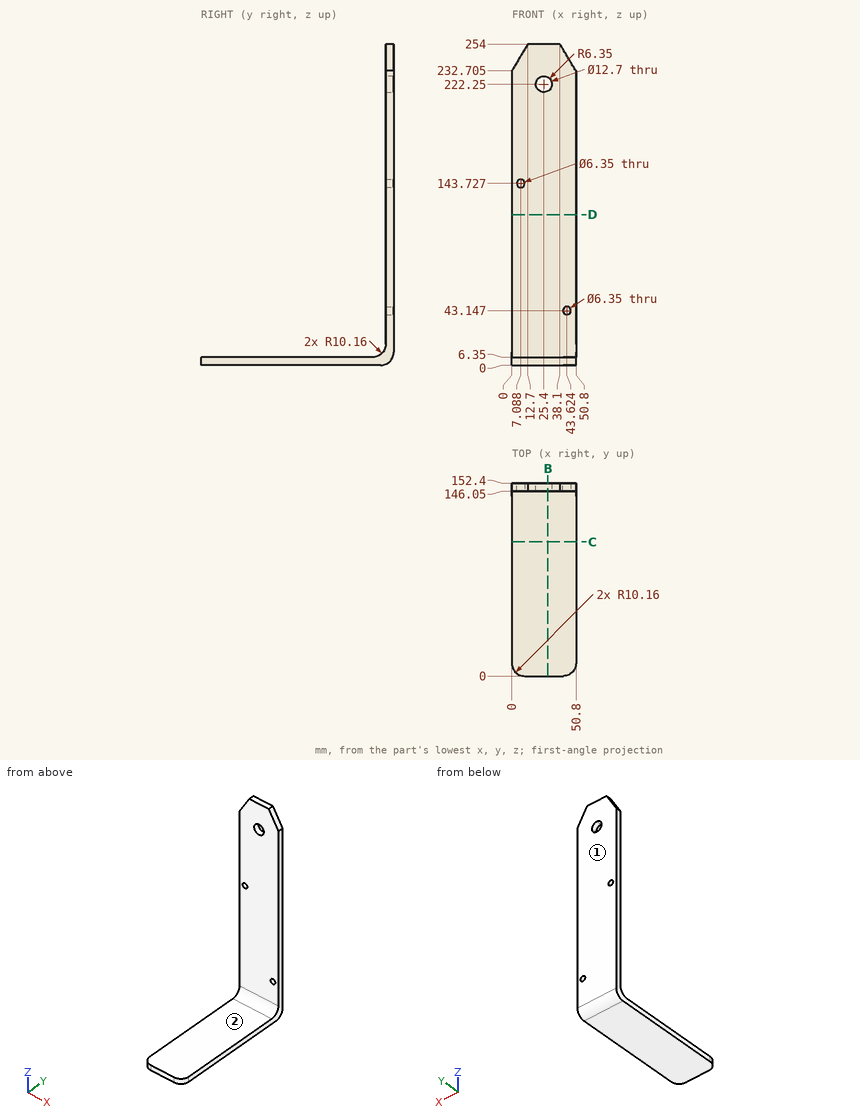
For this review, use the dimensioned drawing (mm, ordinates from the lowest corner) and the shaded views. A direction names the side the tool comes from. Coordinates: 2 decimals unless noted, no trailing zeros. Order: outer loops, then holes, each group sorted by start corner. A loop starts at its lowest first (then second) coordinate and runs counter-clockwise, first axis right, second up. Notation, with made-up numbers: (-21.5, -35) - (-8.5, -35) arc R15 cw to (-8.5, -19) - close; hole circle Ø3 at (22, 1.5). An arc over 180 degrees is marked (long way). Answer as a JSON object with one key per item and string values. Group by question number.
1. Clearance check with flat-ended pins moving along their axes: P1, Ø12, axis at x = 18.5, y = 119, coming from the +Z side; P2, Ø1, axis at x = 7, z = 88, coming from the -Y side; P3, Ø2, axis at x = 44, y = 46, coming from the +Z side. State where each tip first meets the part, or that it passes through.
2. For the marked faces 1 and 2, list the 3-axis set-ups (+Z, -Z, +X, -X, +Y, -Y) from which the entire face can be reached by the end or side of a thin tool; tool diameter is ignored.
3. We need section D-D on z = 119. State the section outline as (x, y) points.
4. We need section B-B on x = 28.5. State the section outline as (y, z) points, then the cut area to 3 significant figures.
5. We need section C-C on y = 106. State the section outline as (x, z) points.
6. For probe 1 along X at (y, z) = (151.25, 222.25); probe 2 along Z at (x, y) = (46.5, 84); probe 3 along Y at (x, z) = (34.5, 85), list the stretches that pass through material, from the lowest coordinate up.
Final values:
{
 "1": {"P1": "z = 6.35", "P2": "y = 146.05", "P3": "z = 6.35"},
 "2": {"face 1": "+Z, -Z, +X, -X, +Y", "face 2": "+Z, +X, -X, -Y"},
 "3": {"outline": "(0, 146.05) - (50.8, 146.05) - (50.8, 152.4) - (0, 152.4) - close"},
 "4": {"outline": "(0, 0) - (142.24, 0) arc R10.16 ccw to (152.4, 10.16) - (152.4, 216.71) - (146.05, 216.71) - (146.05, 16.51) arc R10.16 cw to (135.89, 6.35) - (0, 6.35) - close; (146.05, 227.79) - (152.4, 227.79) - (152.4, 254) - (146.05, 254) - close", "area": "2,470 mm²"},
 "5": {"outline": "(0, 0) - (50.8, 0) - (50.8, 6.35) - (0, 6.35) - close"},
 "6": {"probe 1": "0 to 19.05, 31.75 to 50.8", "probe 2": "0 to 6.35", "probe 3": "146.05 to 152.4"}
}
